from build123d import *

# Parameters (mm, degrees)
REVOLUTION001_ANGLE       = -180
PAD015_DEPTH              = 0.4
BODY012_PLACEMENT_ANGLE   = 180
PAD014_DEPTH              = 2.4
FUSION002_PLACEMENT_ANGLE = 120


with BuildPart() as light001:
    # Sketch024 (on Face1 of ShapeBinder003) → Revolution001 (revolve)
    with BuildSketch(Plane.XY.offset(2.4)):
        with BuildLine():
            ThreePointArc((-2.75, 0), (0, -2.75), (2.75, 0))
            Line((-2.75, 0), (2.75, 0))
        make_face()
    revolve(axis=Axis((-2.75, 0, 2.4), (1, 0, 0)), revolution_arc=REVOLUTION001_ANGLE)


with BuildPart() as body012:
    # Sketch025 (on Face1 of ShapeBinder004) → Pad015 (new body)
    with BuildSketch(Plane(origin=(0, 0, 0), x_dir=(1, 0, 0), z_dir=(0, 0, -1))):
        with BuildLine():
            Line((3.65, 1.5), (6.65, 1.5))
            Line((6.65, 1.5), (6.65, 2))
            Line((6.65, 2), (8.65, 2))
            Line((8.65, 2), (8.65, 0.2))
            Line((8.65, 0.2), (6.65, 0.2))
            Line((6.65, 0.2), (6.65, 0.7))
            Line((6.65, 0.7), (4.45, 0.7))
            Line((4.45, 0.7), (4.45, -0.2))
            ThreePointArc((4.45, -0.2), (3.8, -0.85), (4.45, -1.5))
            Line((4.45, -1.5), (-6.65, -1.5))
            Line((-6.65, -1.5), (-6.65, -1.85))
            Line((-6.65, -1.85), (-8.65, -1.85))
            Line((-8.65, -1.85), (-8.65, -0.25))
            Line((-8.65, -0.25), (-6.65, -0.25))
            Line((-6.65, -0.25), (-6.65, -0.6))
            Line((-6.65, -0.6), (-4.95, -0.6))
            Line((-4.95, -0.6), (-4.95, 1.5))
            Line((-4.95, 1.5), (3.65, 1.5))
        make_face()
    extrude(amount=-PAD015_DEPTH)


with BuildPart() as body012_1:
    # Body012 placement: moved
    add(body012.part.moved(Location((0, 0, 1.4))).rotate(Axis((0, 0, 1.4), (1, 0, 0)), BODY012_PLACEMENT_ANGLE))


with BuildPart() as led2:
    # Sketch023 → Pad014 (new body)
    with BuildSketch(Plane.XY):
        with BuildLine():
            Line((-3.65, 1.75), (-3.65, -1.75))
            ThreePointArc((-3.65, -1.75), (0, -4), (3.65, -1.75))
            Line((3.65, 1.75), (3.65, -1.75))
            ThreePointArc((3.65, 1.75), (0, 4), (-3.65, 1.75))
        make_face()
    extrude(amount=PAD014_DEPTH)

    # Fusion002: union light001, Body012
    add(light001.part)
    add(body012_1.part)


with BuildPart() as led2_1:
    # Fusion002 placement: moved
    add(led2.part.moved(Location((-43, 14, -1.5))).rotate(Axis((-43, 14, -1.5), (0, 0, 1)), FUSION002_PLACEMENT_ANGLE))


solid = led2_1.part
Build history of the part. All positions in model axes, mm. A direction names the side the tool comes from. Round coordinates to 2 decimals unless told otherwise and drop trailing zeros. Write each loop counter-clockwise with the first axis right and the second up, starting at its lowest first coordinate (ties: lowest second). Pieces come first, ordered by that corner, then holes. Notation, with made-up numbers: M 19,17 L 42,17 A21 ccw 42,52 Z; hole C 32,44.25 d8. An arc over 180 degrees is marked long. Answer as a JSON object with one key per item and string values. Group by question number.
(1) Flat gauge pins, fed straight in: pin 1 (1.5 mm diameter, centred on x = -47, y = 18.5, fed in from +Z); pin 2 (2.5 mm diameter, centred on x = -46, y = 19, fed in from -Z); pin 3 (1 mm diameter, centred on y = 9, z = 2.5, fed in from -X); pin 4 (2 mm diameter, centred on y = 16, z = 2, fed in from -X). Where does each tip first touch, or does it go through?
(2) Drill centre lines: L1, parallel to Y at x = -42.75, z = 2.4; L2, parallel to Y at x = -46.5, z = 0.5; L3, parallel to X at y = 17, z = 0.85. Where is each one in solid material? Low to high.
(3) Cut at A-A (y = 18.25). Give the cut face in (x, z).
(4) Which spindle directions (+Z, -Z, +X, -X, +Y, -Y) get a long thin tool onto all of the face, cutting with end or side? Do faces 5 (the flat face through (-40.902, 9.496, -0.297)), 6 (the flat face through (-37.58, 8.31, -0.3)), 7 (the flat face through (-39.4, 9.6, -0.5)), 8 (the flat face through (-47, 19, -0.5)), 9 (the flat face through (-39.4, 9.6, -0.1)). Say none if no direction does.
(5) Cut at D-D (y = 14.25). Give the cut face in (x, z).
(6) Cut at B-B (z = 0.3). Give the cut face in (x, y), and give its area (3 significant figures).
(7) Cut at C-C (y = 10.75). Give the cut face in (x, z), and give its area (3 significant figures).
(8) Mould opens along X. For faces 1 (the flat face through (-47, 19, -0.1)), 2 (the flat face through (-46.39, 18.47, -0.3)), 3 (the flat face through (-48.55, 19.61, -0.3)), 4 (the flat face through (-39.574, 9.267, -0.297)) say: pulls with the +X half, pulls with the -X half, needs draft (parallel to the pull), parting line crosses it, or undercut.
Responses:
{
 "1": {"pin 1": "stops at z = -0.1", "pin 2": "stops at z = -0.5", "pin 3": "passes through", "pin 4": "stops at x = -45.43"},
 "2": {"L1": "y = 11.71 to 16.29", "L2": "y = 12.06 to 16.02", "L3": "x = -45.1 to -40.35"},
 "3": {"outline": "M -47.19,-0.5 L -46.26,-0.5 L -46.26,-0.1 L -47.19,-0.1 Z; M -43.84,-0.5 L -43.72,-0.5 L -43.72,-0.1 L -43.84,-0.1 Z"},
 "4": {"face 5": "+Z, -Z, -Y", "face 6": "+Z, -Z, +X, +Y", "face 7": "-Z, +X, -Y", "face 8": "-Z, -X, +Y", "face 9": "+Z, +X, -Y"},
 "5": {"outline": "M -47.01,-1.5 L -39,-1.5 L -39,0.9 L -40.26,0.9 A2.74 ccw -45.74,0.9 L -47.01,0.9 Z"},
 "6": {"outline": "M -46.34,16.29 A4.09 ccw -42.69,9.96 L -39.66,11.71 A4.09 ccw -43.31,18.04 Z", "area": "49.0 mm2"},
 "7": {"outline": "M -45.34,-1.5 L -41.33,-1.5 L -41.33,-0.5 L -39.39,-0.5 L -39.39,-0.1 L -41.33,-0.1 L -41.33,0.9 L -45.34,0.9 Z", "area": "10.4 mm2"},
 "8": {"face 1": "needs draft", "face 2": "undercut", "face 3": "pulls with the -X half", "face 4": "undercut"}
}
